from build123d import *

# Parameters (mm, degrees)
CARRIER_FRONT_START = 55.5
SKETCH_1_R          = 60
SKETCH_1_R_2        = 17
CARRIER_FRONT_DEPTH = 3
SKETCH_2_R          = 2.25
THROUGH_HOLES_DEPTH = 100
SKETCH_3_R          = 4
CUT_EXTRUDE_2_DEPTH = 100


with BuildPart() as part:
    # Эскиз1 → Carrier_front (new body)
    with BuildSketch(Plane.XY.offset(CARRIER_FRONT_START)):
        Circle(SKETCH_1_R)
        Circle(SKETCH_1_R_2, mode=Mode.SUBTRACT)
    extrude(amount=CARRIER_FRONT_DEPTH)

    # Эскиз2 → Through_holes (cut, symmetric)
    with BuildSketch(Plane.XY):
        with Locations((48, 0)):
            Circle(SKETCH_2_R)
        with Locations((0, 48)):
            Circle(SKETCH_2_R)
        with Locations((-48, 0)):
            Circle(SKETCH_2_R)
        with Locations((0, -48)):
            Circle(SKETCH_2_R)
        with Locations((48.296291314, 12.940952255)):
            Circle(SKETCH_2_R)
        with Locations((12.940952255, 48.296291314)):
            Circle(SKETCH_2_R)
        with Locations((-35.355339059, 35.355339059)):
            Circle(SKETCH_2_R)
        with Locations((-48.296291314, -12.940952255)):
            Circle(SKETCH_2_R)
        with Locations((-12.940952255, -48.296291314)):
            Circle(SKETCH_2_R)
        with Locations((35.355339059, -35.355339059)):
            Circle(SKETCH_2_R)
    extrude(amount=THROUGH_HOLES_DEPTH, both=True, mode=Mode.SUBTRACT)

    # Эскиз3 → Вырез-Вытянуть2 (cut, symmetric)
    with BuildSketch(Plane.XY):
        with Locations((48, 0)):
            Circle(SKETCH_3_R)
        with Locations((0, 48)):
            Circle(SKETCH_3_R)
        with Locations((-48, 0)):
            Circle(SKETCH_3_R)
        with Locations((0, -48)):
            Circle(SKETCH_3_R)
    extrude(amount=CUT_EXTRUDE_2_DEPTH, both=True, mode=Mode.SUBTRACT)


solid = part.part
The model under review builds one solid part; all positions refer to its coordinate system, in mm. Give positions to 0.01 mm unless a question says otherwise; leave off trailing zeros. Write each loop counter-clockwise with the first axis right and the second up, starting at its lowest first coordinate (ties: lowest second). Pieces come first, ordered by that corner, then holes. Notation, with made-up numbers: M -27,-8 L 23,-8 A13 ccw 23,-3 Z; hole C 17,49.25 d9. An arc over 180 degrees is marked long. One line per question, with ' | ' between items. Start each with the question number.
Item 1: For pin 1 (6 mm diameter, centred on x = -48.3, y = -12.94, fed in from +Z); pin 2 (5 mm diameter, centred on x = 48, y = 0, fed in from +Z), all flat-tipped, find the tip position at first contact; note any pin that passes through.
Item 2: We need section A-A on y = 0. Write out the cut boundary in (x, z).
Item 3: Draft analysis for pull direction Y (two halves, no side actions). For faces 1 (the flat face through (12.5, -12.5, 55.5)), 2 (the cylindrical face through (-59.94, 2.64, 56.98)), 3 (the cylindrical face through (44, 0, 57)), state which applies: released by +Y, released by -Y, zero draft, split by the parting line, or undercut.
Item 4: We need section C-C on x = 48. Write out the cut boundary in (y, z).
Item 5: We need section D-D on z = 58. Give the number of separate pieces and of enclosed holes in the cut face, plus the area to 3 significant figures.
Item 6: Wall thickness on line 1 (Y direction, x = -48, z = 56.7); line 2 (Y direction, x = 3.5, z = 57.7); line 3 (X direction, y = 35.5, z = 56.8): over which ranges is each line inside the solid? List them lowest first. Write a range as from..to.
Results found:
1) pin 1: stops at z = 58.5 | pin 2: passes through
2) outline: M -60,55.5 L -52,55.5 L -52,58.5 L -60,58.5 Z; M -44,55.5 L -17,55.5 L -17,58.5 L -44,58.5 Z; M 17,55.5 L 44,55.5 L 44,58.5 L 17,58.5 Z; M 52,55.5 L 60,55.5 L 60,58.5 L 52,58.5 Z
3) face 1: zero draft | face 2: split by the parting line | face 3: undercut
4) outline: M -36,55.5 L -4,55.5 L -4,58.5 L -36,58.5 Z; M 4,55.5 L 10.71,55.5 L 10.71,58.5 L 4,58.5 Z; M 15.17,55.5 L 36,55.5 L 36,58.5 L 15.17,58.5 Z
5) separate pieces: 1 | enclosed holes: 11 | area: 10,100 mm2
6) line 1: y = -36..-15.17, -10.71..-4, 4..36 | line 2: y = -59.9..-49.94, -46.06..-16.64, 16.64..46.06, 49.94..59.9 | line 3: x = -48.37..-37.6, -33.11..48.37
